from build123d import *

# Parameters (mm, degrees)
SKETCH1_W           = 129
SKETCH1_H           = 18
SKETCH1_W_2         = 125.2
SKETCH1_H_2         = 14.45
BOSS_EXTRUDE1_DEPTH = 3
SKETCH2_W           = 129
SKETCH2_H           = 18
BOSS_EXTRUDE2_DEPTH = 3
SKETCH4_R           = 0.81
CUT_EXTRUDE1_DEPTH  = 4
SKETCH5_W           = 30
SKETCH5_H           = 30
SKETCH5_R           = 1.5
BOSS_EXTRUDE4_DEPTH = 3


with BuildPart() as part:
    # Sketch1 → Boss-Extrude1 (new body)
    with BuildSketch(Plane(origin=(0, 0, 0), x_dir=(1, 0, 0), z_dir=(0, 1, 0))):
        Rectangle(SKETCH1_W, SKETCH1_H)
        Rectangle(SKETCH1_W_2, SKETCH1_H_2, mode=Mode.SUBTRACT)
    extrude(amount=BOSS_EXTRUDE1_DEPTH)

    # Sketch2 → Boss-Extrude2 (add)
    with BuildSketch(Plane.XZ):
        Rectangle(SKETCH2_W, SKETCH2_H)
    extrude(amount=BOSS_EXTRUDE2_DEPTH)

    # Sketch4 → Cut-Extrude1 (cut, through all)
    with BuildSketch(Plane(origin=(0, 0, 0), x_dir=(1, 0, 0), z_dir=(0, 1, 0))):
        with Locations((27.97, 0.725)):
            Circle(SKETCH4_R)
        with Locations((-28.08, 0)):
            Circle(SKETCH4_R)
    extrude(amount=-CUT_EXTRUDE1_DEPTH, mode=Mode.SUBTRACT)

    # Sketch5 → Boss-Extrude4 (add)
    with BuildSketch(Plane.XZ.offset(3)):
        with Locations((0, -24)):
            Rectangle(SKETCH5_W, SKETCH5_H)
        with Locations((7.75, -16.092702878)):
            Circle(SKETCH5_R, mode=Mode.SUBTRACT)
        with Locations((7.749201838, -31.592702857)):
            Circle(SKETCH5_R, mode=Mode.SUBTRACT)
        with Locations((-7.75, -31.75)):
            Circle(SKETCH5_R, mode=Mode.SUBTRACT)
        with Locations((-7.749201838, -16.250000021)):
            Circle(SKETCH5_R, mode=Mode.SUBTRACT)
    extrude(amount=-BOSS_EXTRUDE4_DEPTH)


solid = part.part
The listing builds one solid part. Answer for the finished solid, in the listing's coordinates (mm). A direction names the side the tool comes from. Give positions to 0.01 mm unless a question says otherwise; leave off trailing zeros. Write each loop counter-clockwise with the first axis right and the second up, starting at its lowest first coordinate (ties: lowest second). Pieces come first, ordered by that corner, then holes. Notation, with made-up numbers: (22.5, 69) -> (68.5, 69) arc R15 cw to (68.5, 90) -> close; hole circle Ø6 at (-23, -27). An arc over 180 degrees is marked (long way). One line per question, with ' | ' between items. Start each with the question number.
1. Section D-D (z = -13) is taken. Determine the outline of the cut face in (x, y), plus the area to 3 significant figures.
2. Section C-C (x = 11.5) is taken. Determine the outline of the cut face in (y, z) (3 decimals).
3. Section B-B (x = 42) is taken. Determine the outline of the cut face in (y, z) (3 decimals).
4. Find the intervals of material crossed by probe 1 along Z at (x, y) = (7.75, -0.95); probe 2 along Z at (x, y) = (-12, 0.7) (3 decimals); probe 3 along X at (y, z) = (2.4, -6), in increasing order.
5. For faces 1 (the flat face through (-1, 1, -9)), 2 (the flat face through (-15, -2, -24)), 3 (the flat face through (-62.6, 1, 0)), 4 (the flat face through (0, 0, -24)), determine the directions among +Z, -Z, +X, -X, +Y, -Y from which every point of the face is accessible in a straight line to the end or side of a thin tool.
6. Given pin 1 Ø3.5 at (x, y) = (19, 2) entering from -Z; pin 2 Ø2.5 at (x, z) = (-7.75, -31.75) entering from -Y; pin 3 Ø3.5 at (y, z) = (-1, -31) entering from +X; pin 4 Ø1 at (y, z) = (-2, -11.5) entering from -X, each flat-ended and moving along its own axis, determine where each tip first touches the part or whether it passes through.
7. Section A-A (y = 2.05) is taken. Determine the outline of the cut face in (x, z) (3 decimals), plus the area to 3 significant figures.
8. For a pull along Z with two mould halves and no side action, classify faces 5 (the flat face through (-1, 0, 9)), 6 (the flat face through (-1, 1, -7.225)), 7 (the flat face through (0, -2, -39)), 8 (the flat face through (15, -2, -24)) as pulls with the +Z half, pulls with the -Z half, needs draft (parallel to the pull), parting line crosses it, or undercut.
Response values:
1) outline: (-15, -3) -> (15, -3) -> (15, 0) -> (-15, 0) -> close | area: 90.0 mm2
2) outline: (-3, -39) -> (0, -39) -> (0, -9) -> (3, -9) -> (3, -7.225) -> (0, -7.225) -> (0, 7.225) -> (3, 7.225) -> (3, 9) -> (-3, 9) -> close
3) outline: (-3, -9) -> (3, -9) -> (3, -7.225) -> (0, -7.225) -> (0, 7.225) -> (3, 7.225) -> (3, 9) -> (-3, 9) -> close
4) probe 1: -39 to -33.09, -30.09 to -17.59, -14.59 to 9 | probe 2: -9 to -7.225, 7.225 to 9 | probe 3: -64.5 to -62.6, 62.6 to 64.5
5) face 1: -Z, +Y | face 2: -Z, -X, +Y, -Y | face 3: +Y | face 4: -Z, +X, -X, +Y
6) pin 1: z = -9 | pin 2: through | pin 3: x = 15 | pin 4: x = -15
7) outline: (-64.5, -9) -> (64.5, -9) -> (64.5, 9) -> (-64.5, 9) -> close; hole (-62.6, -7.225) -> (62.6, -7.225) -> (62.6, 7.225) -> (-62.6, 7.225) -> close | area: 513 mm2
8) face 5: pulls with the +Z half | face 6: undercut | face 7: pulls with the -Z half | face 8: needs draft
